Autodesk Inventor part; units mm, degrees
ref_plane "Work Plane1" through (0, -862.1118, 0) normal (0, 0, 1) x (-1, 0, 0)
ref_plane "YZ Plane" through (0, 0, 0) normal (1, 0, 0) x (0, 1, 0)
ref_plane "XZ Plane" through (0, 0, 0) normal (0, 1, 0) x (-1, 0, 0)
ref_plane "Work Plane1" through (0, -862.1118, 0) normal (0, 0, 1) x (-1, 0, 0)
sketch "Sketch1" plane through (0, -862.1118, 0) normal (0, 0, 1) x (-1, 0, 0)
  circle A0 centre (-188, -18) radius 4
  line L0 (-220, -478) -> (-220, 22)
  line L1 (-220, -478) -> (-208, -478)
  line L2 (-208, 22) -> (-208, -478)
  line L3 (-220, 22) -> (-208, 22)
  line L4 (-208, -29.2209) -> (-198, -29.2209)
  line L5 (-198, -109.2209) -> (-208, -109.2209)
  line L6 (-208, -109.2209) -> (-208, -29.2209)
  line L7 (-158, -47.7209) -> (-198, -47.7209)
  line L8 (-198, -90.7209) -> (-158, -90.7209)
  line L9 (-158, -90.7209) -> (-158, -47.7209)
  circle A1 centre (-179.15, -68.8709) radius 11.5
  circle A2 centre (-164, -53.7209) radius 2
  circle A3 centre (-195, -53.7209) radius 2
  circle A4 centre (-195, -84.7209) radius 2
  circle A5 centre (-164, -84.7209) radius 2
  line L10 (-195, -84.7209) -> (-195, -53.7209) construction
  line L11 (-195, -84.7209) -> (-164, -84.7209) construction
  line L12 (-198, -29.2209) -> (-198, -47.7209)
  line L13 (-198, -90.7209) -> (-198, -109.2209)
  point P0 (0, -862.1118)
  dimension "d0" = 10
  dimension "d1" = 80
  dimension "d3" = 43
  dimension "d4" = 18.5
  dimension "d5" = 18.5
  dimension "d6" = 23
  dimension "d7" = 4
  dimension "d8" = 4
  dimension "d9" = 4
  dimension "d10" = 4
  dimension "d11" = 31
  dimension "d12" = 31
  dimension "d13" = 31
  dimension "d14" = 31
  dimension "d15" = 6
  dimension "d18" = 6
  dimension "d19" = 6
  dimension "d20" = 6
  dimension "d21" = 90
  dimension "d25" = 21.15
  dimension "d26" = 21.15
  dimension "d27" = 90
  dimension "d28" = 90
  dimension "d29" = 18.5
  dimension "d41" = 40
  dimension "d42" = 40
extrude "Tykkelse" add sketch "Sketch1" along normal blind 20 contours L2 L4 L12 L7 L9 L8 L13 L5
sketch "Sketch2" plane through (198, -832.8909, 0) normal (-1, 0, 0) x (0, 0, 1)
  line L0 (0, 0) -> (20, 0)
  line L1 (20, 18.5) -> (20, 0)
  line L2 (0, 80) -> (0, 61.5)
  line L3 (0, 61.5) -> (20, 61.5)
  line L4 (20, 80) -> (20, 61.5)
  line L5 (0, 80) -> (20, 80)
  circle A0 centre (10, 70) radius 3.5
  circle A1 centre (10, 10) radius 3.5
  point P0 (0, 832.8909)
  dimension "d32" = 7
  dimension "d33" = 7
  dimension "d34" = 10
  dimension "d35" = 10
  dimension "d36" = 10
  dimension "d37" = 10
extrude "Befæstelseshuller" cut sketch "Sketch2" against normal up to surface (10 mm away) contours A0 | A1
fillet "Fillet1" radius 0.5 8 edges at (198, -814.3909, 10) (198, -771.3909, 10) (158, -771.3909, 10) (158, -814.3909, 10) (198, -832.8909, 10) (208, -832.8909, 10) (198, -752.8909, 10) (208, -752.8909, 10)
equation "\"d4\" = d5"
equation "\"d8\" = d7"
equation "\"d9\" = d7"
equation "\"d10\" = d7"
equation "\"d13\" = d11"
equation "\"d14\" = d12"
equation "\"d15\" = d20"
equation "\"d18\" = d15"
equation "\"d19\" = d18"
equation "\"d42\" = d41"
properties part number "Stepper Holder X&Y_2" material "Aluminum 6061"
The model under review builds one solid part; all positions refer to its coordinate system, in mm. A direction names the side the tool comes from. Coordinates: 2 decimals unless noted, no trailing zeros. Write each loop counter-clockwise with the first axis right and the second up, starting at its lowest first coordinate (ties: lowest second). Pieces come first, ordered by that corner, then holes. Notation, with made-up numbers: (17.5, 65) -> (42.5, 65) arc R3 ccw to (42.5, 69) -> close; hole circle Ø4 at (52.25, 27). An arc over 180 degrees is marked (long way). Answer in a Markdown table with one row per item.
1. For faces 1 (the flat face through (208, -793, 10)), 2 (the flat face through (178, -814.391, 10)), 3 (the flat face through (178, -771.391, 10)), list the 3-axis set-ups (+Z, -Z, +X, -X, +Y, -Y) from which the entire face can be reached by the end or side of a thin tool; tool diameter is ignored.
Answers below:
| item | result |
|---|---|
| face 1 | +Z, -Z, +X, +Y, -Y |
| face 2 | +Z, -Z, -X, -Y |
| face 3 | +Z, -Z, -X, +Y |
2. We need section A-A, the plane x = 179.15. State the section outline as (y, z) points.
Answers below:
| item | result |
|---|---|
| outline | (-814.39, 0) -> (-804.74, 0) -> (-804.74, 20) -> (-814.39, 20) -> close; (-781.74, 0) -> (-771.39, 0) -> (-771.39, 20) -> (-781.74, 20) -> close |
3. We need section D-D, the plane y = -822. State the section outline as (x, z) points.
Answers below:
| item | result |
|---|---|
| outline | (198, 0) -> (208, 0) -> (208, 6.62) -> (198, 6.62) -> close; (198, 13.38) -> (208, 13.38) -> (208, 20) -> (198, 20) -> close |
4. Draft analysis for pull direction Z (two halves, no side actions). For faces 4 (the flat face through (198, -826, 8)), 5 (the cylindrical face through (202.93, -759.42, 9.54)), 6 (the flat face through (194, -793, 20)), state which applies: +Z half, -Z half, draft (parallel to the pull), parting line (faces both ways), or undercut.
Answers below:
| item | result |
|---|---|
| face 4 | draft |
| face 5 | undercut |
| face 6 | +Z half |
5. We need section C-C, the plane z = 10. Give the number of separate pieces and of enclosed holes in the cut face, and give its area (3 significant figures).
Answers below:
| item | result |
|---|---|
| separate pieces | 3 |
| enclosed holes | 5 |
| area | 1,910 mm^2 |
6. Wall thickness on probe 1 along Y at (x, z) = (195, 7.25); probe 2 along X at (y, z) = (-808.5, 12.25); probe 3 along Y at (x, z) = (179.15, 6.75): over which ranges is each line inside the solid? List them lowest first. Write a range as [from, to].
Answers below:
| item | result |
|---|---|
| probe 1 | y = [-814.39, -810.39], [-806.39, -779.39], [-775.39, -771.39] |
| probe 2 | x = [158, 162], [166, 193], [197, 208] |
| probe 3 | y = [-814.39, -804.74], [-781.74, -771.39] |
7. Clearance check with flat-ended pins moving along their axes: pin 1 Ø9 at (y, z) = (-822.89, 10) entering from -X; pin 2 Ø1 at (x, z) = (165.5, 3) entering from -Y; pin 3 Ø3 at (x, z) = (173, 10.5) entering from +Y. State where each tip first meets the part, or that it passes through.
Answers below:
| item | result |
|---|---|
| pin 1 | stops at x = 198 |
| pin 2 | stops at y = -814.39 |
| pin 3 | stops at y = -771.39 |
8. We need section B-B, the plane x = 195. State the section outline as (y, z) points.
Answers below:
| item | result |
|---|---|
| outline | (-814.39, 0) -> (-810.39, 0) -> (-810.39, 20) -> (-814.39, 20) -> close; (-806.39, 0) -> (-779.39, 0) -> (-779.39, 20) -> (-806.39, 20) -> close; (-775.39, 0) -> (-771.39, 0) -> (-771.39, 20) -> (-775.39, 20) -> close |
